from build123d import *

# Parameters (mm, degrees)
SKETCH_1_R          = 240
EXTRUDE_1_DEPTH     = 4
SKETCH_2_R          = 2
SKETCH_2_R_2        = 1.5
SKETCH_2_R_3        = 2.5
SKETCH_2_R_4        = 20
CUT_EXTRUDE_2_DEPTH = 340.434824377
CHAMFER_1_SIZE      = 2.5
SKETCH_3_R          = 2
CUT_EXTRUDE_3_DEPTH = 340.434824377
CHAMFER_2_SIZE      = 2


with BuildPart() as part:
    # 草图1 → 凸台-拉伸1 (new body)
    with BuildSketch(Plane(origin=(0, 0, 0), x_dir=(1, 0, 0), z_dir=(0, 1, 0))):
        with Locations(Location((0, 0, 0), (0, 0, 270))):
            Circle(SKETCH_1_R)
    extrude(amount=EXTRUDE_1_DEPTH)

    # 草图2 → 切除-拉伸2 (cut, through all)
    with BuildSketch(Plane(origin=(0, 0, 0), x_dir=(1, 0, 0), z_dir=(0, 1, 0))):
        with Locations(Location((-45.033320997, 26, 0), (0, 0, 270))):
            Circle(SKETCH_2_R)
        with Locations(Location((0, 52, 0), (0, 0, 270))):
            Circle(SKETCH_2_R)
        with Locations(Location((45.033320997, 26, 0), (0, 0, 270))):
            Circle(SKETCH_2_R)
        with Locations(Location((45.033320997, -26, 0), (0, 0, 270))):
            Circle(SKETCH_2_R)
        with Locations(Location((0, -52, 0), (0, 0, 270))):
            Circle(SKETCH_2_R)
        with Locations(Location((-45.033320997, -26, 0), (0, 0, 270))):
            Circle(SKETCH_2_R)
        with Locations(Location((-64.5, 130, 0), (0, 0, 270))):
            Circle(SKETCH_2_R_2)
        with Locations(Location((100, 0, 0), (0, 0, 270))):
            Circle(SKETCH_2_R_3)
        with Locations(Location((100, 60, 0), (0, 0, 270))):
            Circle(SKETCH_2_R_3)
        with Locations(Location((100, 120, 0), (0, 0, 270))):
            Circle(SKETCH_2_R_3)
        with Locations(Location((100, 180, 0), (0, 0, 270))):
            Circle(SKETCH_2_R_3)
        with Locations(Location((100, -60, 0), (0, 0, 270))):
            Circle(SKETCH_2_R_3)
        with Locations(Location((100, -120, 0), (0, 0, 270))):
            Circle(SKETCH_2_R_3)
        with Locations(Location((100, -180, 0), (0, 0, 270))):
            Circle(SKETCH_2_R_3)
        with Locations(Location((-100, -180, 0), (0, 0, 90))):
            Circle(SKETCH_2_R_3)
        with Locations(Location((-100, -120, 0), (0, 0, 90))):
            Circle(SKETCH_2_R_3)
        with Locations(Location((-100, -60, 0), (0, 0, 90))):
            Circle(SKETCH_2_R_3)
        with Locations(Location((-100, 180, 0), (0, 0, 90))):
            Circle(SKETCH_2_R_3)
        with Locations(Location((-100, 120, 0), (0, 0, 90))):
            Circle(SKETCH_2_R_3)
        with Locations(Location((-100, 60, 0), (0, 0, 90))):
            Circle(SKETCH_2_R_3)
        with Locations(Location((-100, 0, 0), (0, 0, 90))):
            Circle(SKETCH_2_R_3)
        with Locations(Location((-50.5, 130, 0), (0, 0, 270))):
            Circle(SKETCH_2_R_2)
        with Locations(Location((-64.5, 110, 0), (0, 0, 270))):
            Circle(SKETCH_2_R_2)
        with Locations(Location((-50.5, 110, 0), (0, 0, 270))):
            Circle(SKETCH_2_R_2)
        with Locations(Location((0, 0, 0), (0, 0, 270))):
            Circle(SKETCH_2_R_4)
        with Locations(Location((170, 90, 0), (0, 0, 270))):
            Circle(SKETCH_2_R)
        with Locations(Location((170, -90, 0), (0, 0, 270))):
            Circle(SKETCH_2_R)
        with Locations(Location((-170, -90, 0), (0, 0, 90))):
            Circle(SKETCH_2_R)
        with Locations(Location((-170, 90, 0), (0, 0, 90))):
            Circle(SKETCH_2_R)
        with Locations(Location((215, -70, 0), (0, 0, 270))):
            Circle(SKETCH_2_R)
        with Locations(Location((215, 70, 0), (0, 0, 90))):
            Circle(SKETCH_2_R)
        with Locations(Location((-215, 70, 0), (0, 0, 270))):
            Circle(SKETCH_2_R)
        with Locations(Location((-215, -70, 0), (0, 0, 90))):
            Circle(SKETCH_2_R)
    extrude(amount=CUT_EXTRUDE_2_DEPTH, mode=Mode.SUBTRACT)

    # 倒角1
    chamfer_1_edges = [part.edges().sort_by_distance(p)[0] for p in [
        (-45.033320997, 4, -28),
        (0, 4, -54),
        (45.033320997, 4, -28),
        (45.033320997, 4, 24),
        (0, 4, 50),
        (-45.033320997, 4, 24),
    ]]
    chamfer(chamfer_1_edges, length=CHAMFER_1_SIZE)

    # 草图3 → 切除-拉伸3 (cut, through all)
    with BuildSketch(Plane(origin=(0, 0, 0), x_dir=(1, 0, 0), z_dir=(0, 1, 0))):
        with Locations(Location((151.880580048, 173.093783484, 0), (0, 0, 270))):
            Circle(SKETCH_3_R)
        with Locations(Location((-15, 229.791576166, 0), (0, 0, 270))):
            Circle(SKETCH_3_R)
        with Locations(Location((-15, 219.791576166, 0), (0, 0, 270))):
            Circle(SKETCH_3_R)
        with Locations(Location((15, 219.791576166, 0), (0, 0, 90))):
            Circle(SKETCH_3_R)
        with Locations(Location((15, 229.791576166, 0), (0, 0, 90))):
            Circle(SKETCH_3_R)
        with Locations(Location((144.809512237, 166.022715672, 0), (0, 0, 270))):
            Circle(SKETCH_3_R)
        with Locations(Location((173.093783484, 151.880580048, 0), (0, 0, 90))):
            Circle(SKETCH_3_R)
        with Locations(Location((166.022715672, 144.809512237, 0), (0, 0, 90))):
            Circle(SKETCH_3_R)
        with Locations(Location((229.791576166, 15, 0), (0, 0, 270))):
            Circle(SKETCH_3_R)
        with Locations(Location((219.791576166, 15, 0), (0, 0, 270))):
            Circle(SKETCH_3_R)
        with Locations(Location((229.791576166, -15, 0), (0, 0, 90))):
            Circle(SKETCH_3_R)
        with Locations(Location((219.791576166, -15, 0), (0, 0, 90))):
            Circle(SKETCH_3_R)
        with Locations(Location((173.093783484, -151.880580048, 0), (0, 0, 270))):
            Circle(SKETCH_3_R)
        with Locations(Location((166.022715672, -144.809512237, 0), (0, 0, 270))):
            Circle(SKETCH_3_R)
        with Locations(Location((151.880580048, -173.093783484, 0), (0, 0, 90))):
            Circle(SKETCH_3_R)
        with Locations(Location((144.809512237, -166.022715672, 0), (0, 0, 90))):
            Circle(SKETCH_3_R)
        with Locations(Location((15, -229.791576166, 0), (0, 0, 270))):
            Circle(SKETCH_3_R)
        with Locations(Location((15, -219.791576166, 0), (0, 0, 270))):
            Circle(SKETCH_3_R)
        with Locations(Location((-15, -229.791576166, 0), (0, 0, 90))):
            Circle(SKETCH_3_R)
        with Locations(Location((-15, -219.791576166, 0), (0, 0, 90))):
            Circle(SKETCH_3_R)
        with Locations(Location((-151.880580048, -173.093783484, 0), (0, 0, 270))):
            Circle(SKETCH_3_R)
        with Locations(Location((-144.809512237, -166.022715672, 0), (0, 0, 270))):
            Circle(SKETCH_3_R)
        with Locations(Location((-173.093783484, -151.880580048, 0), (0, 0, 90))):
            Circle(SKETCH_3_R)
        with Locations(Location((-166.022715672, -144.809512237, 0), (0, 0, 90))):
            Circle(SKETCH_3_R)
        with Locations(Location((-229.791576166, -15, 0), (0, 0, 270))):
            Circle(SKETCH_3_R)
        with Locations(Location((-219.791576166, -15, 0), (0, 0, 270))):
            Circle(SKETCH_3_R)
        with Locations(Location((-229.791576166, 15, 0), (0, 0, 90))):
            Circle(SKETCH_3_R)
        with Locations(Location((-219.791576166, 15, 0), (0, 0, 90))):
            Circle(SKETCH_3_R)
        with Locations(Location((-173.093783484, 151.880580048, 0), (0, 0, 270))):
            Circle(SKETCH_3_R)
        with Locations(Location((-166.022715672, 144.809512237, 0), (0, 0, 270))):
            Circle(SKETCH_3_R)
        with Locations(Location((-151.880580048, 173.093783484, 0), (0, 0, 90))):
            Circle(SKETCH_3_R)
        with Locations(Location((-144.809512237, 166.022715672, 0), (0, 0, 90))):
            Circle(SKETCH_3_R)
        with BuildLine():
            Line((-10, 239.791576166), (-10, 224.791576166))
            Line((-10, 224.791576166), (10, 224.791576166))
            Line((10, 224.791576166), (10, 239.791576166))
            ThreePointArc((10, 239.791576166), (0, 240), (-10, 239.791576166))
        make_face()
        with BuildLine():
            Line((166.022715672, 151.880580048), (176.62931739, 162.487181766))
            ThreePointArc((176.62931739, 162.487181766), (169.705627485, 169.705627485), (162.487181766, 176.62931739))
            Line((162.487181766, 176.62931739), (151.880580048, 166.022715672))
            Line((151.880580048, 166.022715672), (166.022715672, 151.880580048))
        make_face()
        with BuildLine():
            Line((224.791576166, -10), (239.791576166, -10))
            ThreePointArc((239.791576166, -10), (240, 0), (239.791576166, 10))
            Line((239.791576166, 10), (224.791576166, 10))
            Line((224.791576166, 10), (224.791576166, -10))
        make_face()
        with BuildLine():
            Line((151.880580048, -166.022715672), (162.487181766, -176.62931739))
            ThreePointArc((162.487181766, -176.62931739), (169.705627485, -169.705627485), (176.62931739, -162.487181766))
            Line((176.62931739, -162.487181766), (166.022715672, -151.880580048))
            Line((166.022715672, -151.880580048), (151.880580048, -166.022715672))
        make_face()
        with BuildLine():
            Line((-10, -224.791576166), (-10, -239.791576166))
            ThreePointArc((-10, -239.791576166), (0, -240), (10, -239.791576166))
            Line((10, -239.791576166), (10, -224.791576166))
            Line((10, -224.791576166), (-10, -224.791576166))
        make_face()
        with BuildLine():
            Line((-166.022715672, -151.880580048), (-176.62931739, -162.487181766))
            ThreePointArc((-176.62931739, -162.487181766), (-169.705627485, -169.705627485), (-162.487181766, -176.62931739))
            Line((-162.487181766, -176.62931739), (-151.880580048, -166.022715672))
            Line((-151.880580048, -166.022715672), (-166.022715672, -151.880580048))
        make_face()
        with BuildLine():
            Line((-224.791576166, 10), (-239.791576166, 10))
            ThreePointArc((-239.791576166, 10), (-240, 0), (-239.791576166, -10))
            Line((-239.791576166, -10), (-224.791576166, -10))
            Line((-224.791576166, -10), (-224.791576166, 10))
        make_face()
        with BuildLine():
            Line((-151.880580048, 166.022715672), (-162.487181766, 176.62931739))
            ThreePointArc((-162.487181766, 176.62931739), (-169.705627485, 169.705627485), (-176.62931739, 162.487181766))
            Line((-176.62931739, 162.487181766), (-166.022715672, 151.880580048))
            Line((-166.022715672, 151.880580048), (-151.880580048, 166.022715672))
        make_face()
    extrude(amount=CUT_EXTRUDE_3_DEPTH, mode=Mode.SUBTRACT)

    # 倒角2
    chamfer_2_edges = [part.edges().sort_by_distance(p)[0] for p in [
        (170, 0, -92),
        (170, 0, 88),
        (-170, 0, 92),
        (-170, 0, -88),
        (215, 0, 68),
        (215, 0, -68),
        (-215, 0, -72),
        (-215, 0, 72),
    ]]
    chamfer(chamfer_2_edges, length=CHAMFER_2_SIZE)


solid = part.part
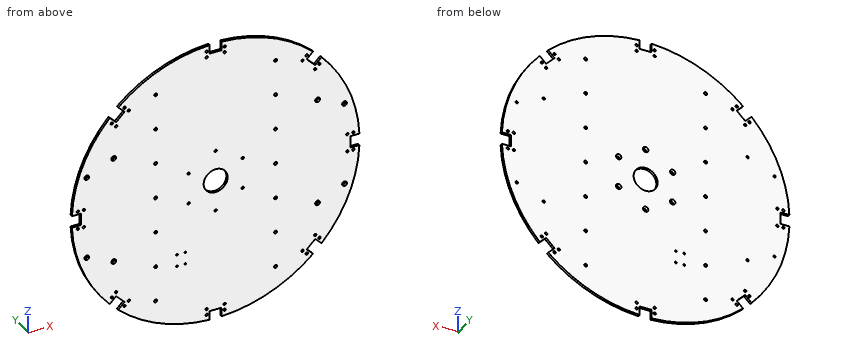
Here's how the part is built. I have some questions about the finished solid (model axes, mm). Give positions to 0.01 mm unless a question says otherwise; leave off trailing zeros. Order: outer loops, then holes, each group sorted by start corner. A loop starts at its lowest first (then second) coordinate and runs counter-clockwise, first axis right, second up. Notation, with made-up numbers: M 12.25,72 L 30.25,72 A16 cw 30.25,101 Z; hole C -38.5,17.5 d10. An arc over 180 degrees is marked long. Answer as a JSON object with one key per item and string values. Group by question number.
1) Suppose I cut it at C-C, the plane x = -201.5. Write out the boundary of the cut face in (y, z), plus the area to 3 significant figures.
2) Please list where these lines run through material, in increasing order: L1, parallel to Z at x = -215, y = 1.15; L2, parallel to X at y = 3.25, z = -60; L3, parallel to Z at x = 15, y = 1.1. Write a range as [from, to].
3) Suppose I cut it at B-B, the plane z = 204. Write out the boundary of the cut face in (x, y).
4) Suppose I cut it at A-A, the plane y = 2.65. Count the separate pieces of the cut face and the enclosed holes in it, plus the area to 3 significant figures.
Results found:
{
 "1": {"outline": "M 0,-130.38 L 4,-130.38 L 4,130.38 L 0,130.38 Z", "area": "1,040 mm²"},
 "2": {"L1": "[-106.65, -72.85], [-67.15, 67.15], [72.85, 106.65]", "L2": "[-232.38, -102.5], [-97.5, 97.5], [102.5, 232.38]", "L3": "[-239.53, -231.79], [-227.79, -221.79], [-217.79, -13.23], [13.23, 217.79], [221.79, 227.79], [231.79, 239.53]"},
 "3": {"outline": "M -126.43,0 L 126.43,0 L 126.43,4 L -126.43,4 Z"},
 "4": {"separate pieces": "1", "enclosed holes": "65", "area": "176,000 mm²"}
}
